from build123d import *

# Parameters (mm, degrees)
F0_W     = 100
F0_H     = 100
F1_DEPTH = 42
F2_W     = 56.480739
F2_H     = 58.809845
F3_DEPTH = 48.7
F4_R     = 15.824567
F5_DEPTH = 73.9
F6_DEPTH = 25


with BuildPart() as f1:
    # F0 (on Top) → F1 (new body)
    with BuildSketch(Plane.XY):
        with Locations((-0.727845, -2.89979)):
            Rectangle(F0_W, F0_H)
    extrude(amount=F1_DEPTH)

    # F2 (on face) → F3 (join)
    with BuildSketch(Plane.XY.offset(42)):
        with Locations((2.183533, 7.569583)):
            Rectangle(F2_W, F2_H)
    extrude(amount=F3_DEPTH)

    # F4 (on face) → F5 (join)
    with BuildSketch(Plane.XY.offset(90.7)):
        with Locations((0, 3.947993)):
            Circle(F4_R)
    extrude(amount=F5_DEPTH)

    # F0 (on Top) → F6 (join)
    with BuildSketch(Plane.XY):
        with Locations((-0.727845, -2.89979)):
            Rectangle(F0_W, F0_H)
    extrude(amount=F6_DEPTH)


solid = f1.part
Verification items for the finished model (mm, model axes). A direction names the side the tool comes from. Coordinates: 2 decimals unless noted, no trailing zeros. Order: outer loops, then holes, each group sorted by start corner. A loop starts at its lowest first (then second) coordinate and runs counter-clockwise, first axis right, second up.
1. Sectioned sample at D-D, the plane x = 28. Record the cut outline in (y, z), and give its area (3 significant figures).
Results found:
outline: (-52.9, 0) - (47.1, 0) - (47.1, 42) - (36.97, 42) - (36.97, 90.7) - (-21.84, 90.7) - (-21.84, 42) - (-52.9, 42) - close
area: 7,060 mm2
2. Sectioned sample at C-C, the plane z = 66. Record the cut outline in (x, y), and give its area (3 significant figures).
Results found:
outline: (-26.06, -21.84) - (30.42, -21.84) - (30.42, 36.97) - (-26.06, 36.97) - close
area: 3,320 mm2
3. Set-up check for faces 1 (the face through (-26.057, 7, 66)), 2 (the face through (30.424, 7, 66)), 3 (the face through (2, -21.835, 66)), 4 (the face through (2, 21, 90.7)), 5 (the face through (2, 36.975, 66)): record each of +Z, -Z, +X, -X, +Y, -Y from which the full face is reachable in a straight line by a thin tool's end or side.
Results found:
face 1: +Z, -X, +Y, -Y
face 2: +Z, +X, +Y, -Y
face 3: +Z, +X, -X, -Y
face 4: +Z
face 5: +Z, +X, -X, +Y
4. Sectioned sample at B-B, the plane y = -15. Record the cut outline in (x, z).
Results found:
outline: (-50.73, 0) - (49.27, 0) - (49.27, 42) - (30.42, 42) - (30.42, 90.7) - (-26.06, 90.7) - (-26.06, 42) - (-50.73, 42) - close
5. Sectioned sample at A-A, the plane x = 0. Record the cut outline in (y, z).
Results found:
outline: (-52.9, 0) - (47.1, 0) - (47.1, 42) - (36.97, 42) - (36.97, 90.7) - (19.77, 90.7) - (19.77, 164.6) - (-11.88, 164.6) - (-11.88, 90.7) - (-21.84, 90.7) - (-21.84, 42) - (-52.9, 42) - close
6. Go/stop test with flat-tipped pins: pin 1 Ø5 at (x, y) = (1.5, -22.5) entering from +Z; pin 2 Ø10 at (x, y) = (34, -17) entering from -Z; pin 3 Ø4 at (x, z) = (2.5, 77.5) entering from -Y; pin 4 Ø3 at (x, y) = (-36, -30) entering from +Z. Record where each tip stops, or that it passes through.
Results found:
pin 1: stops at z = 90.7
pin 2: stops at z = 0
pin 3: stops at y = -21.84
pin 4: stops at z = 42
7. Scan lines: line 1 (Z direction, x = -40.5, y = 9.5); line 2 (Y direction, x = -17, z = 51.5); line 3 (X direction, y = -4.5, z = 86). Record each from-to range of solid material in increasing order.
Results found:
line 1: z = 0 to 42
line 2: y = -21.84 to 36.97
line 3: x = -26.06 to 30.42
